Autodesk Inventor part; units mm, degrees
ref_plane "YZ Plane" through (0, 0, 0) normal (1, 0, 0) x (0, 1, 0)
ref_plane "XZ Plane" through (0, 0, 0) normal (0, 1, 0) x (-1, 0, 0)
ref_plane "XY Plane" through (0, 0, 0) normal (0, 0, 1) x (1, 0, 0)
sketch "Sketch1" plane through (0, 0, 0) normal (0, 1, 0) x (-1, 0, 0)
  line L0 (0, 0) -> (-25.4, 0)
  line L1 (-25.4, 0) -> (-25.4, -3.81)
  line L2 (-25.4, -3.81) -> (0, -3.81)
  line L3 (0, -3.81) -> (0, 0)
  line L4 (-25.4, 0) -> (-21.59, 0)
  line L5 (-21.59, 0) -> (-21.59, -25.4)
  line L6 (-21.59, -25.4) -> (-25.4, -25.4)
  line L7 (-25.4, -25.4) -> (-25.4, 0)
  dimension "d0" = 25.4
  dimension "d1" = 3.81
  dimension "d2" = 3.81
  dimension "d3" = 25.4
extrude "Extrusion1" add sketch "Sketch1" along normal blind 22.86
sketch "Sketch2" plane through (21.59, 0, -25.4) normal (-1, 0, 0) x (0, 0, 1)
  line L0 (0, 0) -> (0, 22.86)
  line L1 (0, 11.43) -> (10.795, 11.43)
  point P0 (25.4, 0)
  dimension "d9" = 10.795
hole "Hole1" at (21.59, 11.43, -14.605) direction (1, 0, 0) diameter 2.794 end through all
sketch "Sketch3" plane through (21.59, 0, -3.81) normal (0, 0, -1) x (-1, 0, 0)
  line L0 (21.59, 0) -> (21.59, 22.86)
  line L1 (21.59, 11.43) -> (10.795, 11.43)
  dimension "d17" = 10.795
hole "Hole2" at (10.795, 11.43, -3.81) direction (0, 0, 1) diameter 5.08 end through all
properties part number "part v5"
Input: part model. Units: mm. Frame: model coordinates. Round coordinates to 2 decimals unless told otherwise and drop trailing zeros. Order: outer loops, then holes, each group sorted by start corner. A loop starts at its lowest first (then second) coordinate and runs counter-clockwise, first axis right, second up. Notation, with made-up numbers: (13, -0.5) - (47, -0.5) arc R21 cw to (47, 29.5) - close; hole circle Ø5 at (40, 47.5). An arc over 180 degrees is marked (long way). Answer as a JSON object with one key per item and string values. Group by question number.
(1) Cut plane D-D (x = 13.75). Return loops of the section in (y, z), then the cut area to 3 significant figures.
(2) Cut plane A-A (z = -15). Return loops of the section in (x, y).
(3) Pin query (flat end, axial travel): P1, Ø12, axis at x = 14.5, y = 19, coming from the +Z side; P2, Ø3, axis at x = 15.5, y = 8.5, coming from the -Z side; P3, Ø3, axis at y = 9.5, z = -6, coming from the -X side. Return the tip coordinate at first contact, or that it passes through.
(4) Cut plane C-C (y = 7). Return loops of the section in (x, z), then the cut area to 3 significant figures.
(5) Material intervals for probe 1 along Z at (x, y) = (23.55, 11.43); probe 2 along X at (y, z) = (11.43, -1.4) (3 decimals); probe 3 along Z at (x, y) = (21, 3.25), sorted ascending. Write a range as from..to.
(6) Cut plane B-B (y = 11.43). Return loops of the section in (x, z) (3 decimals), then the cut area to 3 significant figures.
(7) Draft query along Z for faces 1 (the face through (21.59, 11, -12)), 2 (the face through (23.522, 11.01, -13.273)), 3 (the face through (10.9, 8.7, -3.81)). Return one class per face: released by +Z, released by -Z, zero draft, split by the parting line, or undercut.
Here are the results:
{
 "1": {"outline": "(0, -3.81) - (22.86, -3.81) - (22.86, 0) - (0, 0) - close", "area": "87.1 mm^2"},
 "2": {"outline": "(21.59, 0) - (25.4, 0) - (25.4, 10.09) - (21.59, 10.09) - close; (21.59, 12.77) - (25.4, 12.77) - (25.4, 22.86) - (21.59, 22.86) - close"},
 "3": {"P1": "stops at z = 0", "P2": "stops at z = -3.81", "P3": "stops at x = 21.59"},
 "4": {"outline": "(0, -3.81) - (21.59, -3.81) - (21.59, -25.4) - (25.4, -25.4) - (25.4, 0) - (0, 0) - close", "area": "179 mm^2"},
 "5": {"probe 1": "z = -25.4..-16, -13.21..0", "probe 2": "x = 0..8.255, 13.335..25.4", "probe 3": "z = -3.81..0"},
 "6": {"outline": "(0, -3.81) - (8.255, -3.81) - (8.255, 0) - (0, 0) - close; (13.335, -3.81) - (21.59, -3.81) - (21.59, -13.208) - (25.4, -13.208) - (25.4, 0) - (13.335, 0) - close; (21.59, -25.4) - (25.4, -25.4) - (25.4, -16.002) - (21.59, -16.002) - close", "area": "149 mm^2"},
 "7": {"face 1": "zero draft", "face 2": "undercut", "face 3": "released by -Z"}
}
